```python
from build123d import *

# Parameters (mm, degrees)
BOSS_EXTRUDE1_DEPTH = 304.8
FILLET1_R           = 1.651


with BuildPart() as part:
    # Sketch1 → Boss-Extrude1 (new body)
    with BuildSketch(Plane.XY):
        Polygon((-4.7625, 1.984375), (-15.060088734, 1.984375), (-15.875, 1.162346283), (-14.702501762, 0), (-13.954431554, 0.754603868), (-13.121373906, 0.197134811), (-3.203280151, 0.197134811), (-2.402359615, 15.414625), (0, 15.414625), (2.402359615, 15.414625), (3.203280151, 0.197134811), (13.121373906, 0.197134811), (13.954431554, 0.754603868), (14.702501762, 0), (15.875, 1.162346283), (15.060088734, 1.984375), (4.7625, 1.984375), (3.96875, 17.065625), (0, 17.065625), (-3.96875, 17.065625), align=None)
    extrude(amount=-BOSS_EXTRUDE1_DEPTH)

    # Fillet1
    fillet1_edges = [part.edges().sort_by_distance(p)[0] for p in [
        (-15.060088734, 1.984375, -152.4),
        (-3.96875, 17.065625, -152.4),
        (3.96875, 17.065625, -152.4),
        (15.060088734, 1.984375, -152.4),
        (3.203280151, 0.197134811, -152.4),
        (-3.203280151, 0.197134811, -152.4),
    ]]
    fillet(fillet1_edges, radius=FILLET1_R)


solid = part.part
```
The listing builds one solid part. Answer for the finished solid, in the listing's coordinates (mm). A direction names the side the tool comes from. Give positions to 0.01 mm unless a question says otherwise; leave off trailing zeros. Order: outer loops, then holes, each group sorted by start corner. A loop starts at its lowest first (then second) coordinate and runs counter-clockwise, first axis right, second up. Notation, with made-up numbers: (-2.5, -38.5) -> (6.5, -38.5) arc R32 ccw to (6.5, -11.5) -> close; hole circle Ø10 at (51, 45.25). An arc over 180 degrees is marked (long way). One line per item, written item: value.
1) A tool of negligible diameter and unlimited length cuts with its end or side. For faces 4 (the flat face through (3.5, 6, 0)), 5 (the flat face through (10, 1.984, -150)), 6 (the flat face through (3.5, 6, -304.8)), 7 (the flat face through (2.757, 8.684, -150.266)), 8 (the flat face through (-9, 1.984, -150)), from which of +Z, -Z, +X, -X, +Y, -Y can it reach the whole face along a straight path? Write none if from no direction.
Reported:
face 4: +Z, +X, -X, +Y, -Y
face 5: +Z, -Z, +X, +Y
face 6: -Z, +X, -X, +Y, -Y
face 7: +Z, -Z, -Y
face 8: +Z, -Z, -X, +Y
2) Find section C-C, the plane x = 7.5. Determine the outline of the cut face in (y, z), plus the area to 3 significant figures.
Reported:
outline: (0.2, -304.8) -> (1.98, -304.8) -> (1.98, 0) -> (0.2, 0) -> close
area: 545 mm^2
3) Find section B-B, the plane y = 4.75. Determine the outline of the cut face in (x, z).
Reported:
outline: (-4.62, -304.8) -> (-2.96, -304.8) -> (-2.96, 0) -> (-4.62, 0) -> close; (2.96, -304.8) -> (4.62, -304.8) -> (4.62, 0) -> (2.96, 0) -> close
4) Find section A-A, the plane z = -74.5. Determine the outline of the cut face in (x, y) (1 decimal).
Reported:
outline: (-15.9, 1.2) -> (-14.7, 0) -> (-14, 0.8) -> (-13.1, 0.2) -> (-4.8, 0.2) arc R1.7 ccw to (-3.1, 1.8) -> (-2.4, 15.4) -> (2.4, 15.4) -> (3.1, 1.8) arc R1.7 ccw to (4.8, 0.2) -> (13.1, 0.2) -> (14, 0.8) -> (14.7, 0) -> (15.9, 1.2) -> (15.5, 1.5) arc R1.7 ccw to (14.4, 2) -> (4.8, 2) -> (4.1, 15.5) arc R1.7 ccw to (2.4, 17.1) -> (-2.4, 17.1) arc R1.7 ccw to (-4.1, 15.5) -> (-4.8, 2) -> (-14.4, 2) arc R1.7 ccw to (-15.5, 1.5) -> close
5) Flat-ended cylindrical pins translate along their axes: P1, Ø10, axis at y = 13, z = -95.5, coming from the +X side; P2, Ø1, axis at y = 9.5, z = -131, coming from the -X side; P3, Ø7.5, axis at x = -10.5, z = -191, coming from the +Y side. Find the tip coordinate at first contact, or state that the pin passes through.
Reported:
P1: stops at x = 4.45
P2: stops at x = -4.39
P3: stops at y = 1.98
6) Find the intervals of material crossed by line 1 (X direction, y = 15, z = -104.5); line 2 (Y direction, x = 13, z = -204); line 3 (Y direction, x = 0.5, z = -187.5), in increasing order.
Reported:
line 1: x = -4.08 to -2.42, 2.42 to 4.08
line 2: y = 0.2 to 1.98
line 3: y = 15.41 to 17.07
7) Determine the mould class of faces 1 (the flat face through (9, 0.197, -150)), 2 (the flat face through (-4.4, 8.84, -150.27)), 3 (the flat face through (0, 17.066, -150)) for opening direction X: pulls with the +X half, pulls with the -X half, needs draft (parallel to the pull), parting line crosses it, or undercut.
Reported:
face 1: undercut
face 2: pulls with the -X half
face 3: needs draft
